Answer from the drawing. Dimensions are ordinates in mm from the lowest x, y and z of the part. Give positions to 0.01 mm unless a question says otherwise; leave off trailing zeros. Loops run counter-clockwise (first coordinate to the right, second up) from the corner with the lowest first, then second, coordinate; pieces in that order, holes last. Notation, with made-up numbers: (43, 47.25) - (90, 47.25) arc R19 ccw to (90, 71.25) - close; hole circle Ø3 at (77, 21.5). An arc over 180 degrees is marked (long way). One line per item, written item: value.
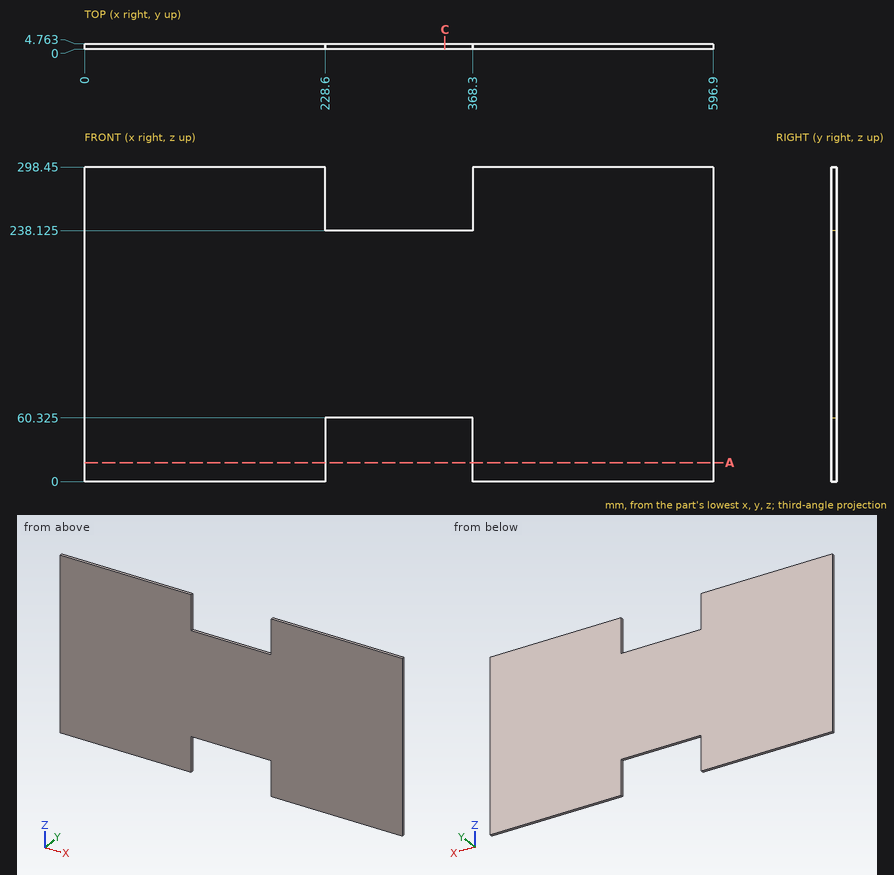
1. A flat-ended cylindrical pin translates along its axis: pin 1 Ø1.4 at (x, y) = (302.5, 3.5) entering from +Z (1 decimal). Find the tip coordinate at first contact, or state that the pin passes through.
Output:
pin 1: stops at z = 238.1
2. Section A-A (z = 18) is taken. Write down the section's boundary in (x, y).
Output:
outline: (0, 0) - (228.6, 0) - (228.6, 4.76) - (0, 4.76) - close; (368.3, 0) - (596.9, 0) - (596.9, 4.76) - (368.3, 4.76) - close
3. Section C-C (x = 342) is taken. Write down the section's boundary in (y, z) (1 decimal).
Output:
outline: (0, 60.3) - (4.8, 60.3) - (4.8, 238.1) - (0, 238.1) - close
4. Find the intervals of material crossed by line 1 along X through (y, z) = (1.6, 28); line 2 along Z through (x, y) = (276, 3.05) (1 decimal), in increasing order.
Output:
line 1: x = 0 to 228.6, 368.3 to 596.9
line 2: z = 60.3 to 238.1
